Autodesk Inventor part; units mm, degrees
ref_plane "YZ Plane" through (0, 0, 0) normal (1, 0, 0) x (0, 1, 0)
ref_plane "XZ Plane" through (0, 0, 0) normal (0, 1, 0) x (-1, 0, 0)
ref_plane "XY Plane" through (0, 0, 0) normal (0, 0, 1) x (1, 0, 0)
sketch "Sketch1" plane through (0, 0, 0) normal (0, 1, 0) x (-1, 0, 0)
  circle A0 centre (0, 0) radius 13.95
  line L0 (-1.48, 13.8713) -> (-1.48, 10.9113) construction
  line L1 (-1.48, 10.9113) -> (1.48, 10.9113) construction
  line L2 (1.48, 10.9113) -> (1.48, 13.8713) construction
  line L3 (1.33, 13.8865) -> (1.33, 11.0613)
  line L4 (1.33, 11.0613) -> (-1.33, 11.0613)
  line L5 (-1.33, 11.0613) -> (-1.33, 13.8865)
  line L6 (-1.33, -13.8865) -> (-1.33, -11.0613)
  line L7 (-1.33, -11.0613) -> (1.33, -11.0613)
  line L8 (1.33, -11.0613) -> (1.33, -13.8865)
  arc A1 (15.7257, 8.6547) -> (8.6547, -15.7257) centre (0, 0) ccw
  line L9 (0, 0) -> (0, -53.8283) construction
  line L10 (0, 0) -> (-28.2843, -28.2843) construction
  line L11 (0, 0) -> (-45.9619, 45.9619) construction
  line L12 (0, 0) -> (-69.2668, 0) construction
  circle A2 centre (-28.2843, -28.2843) radius 3
  circle A3 centre (-45.9619, 45.9619) radius 3
  line L13 (-8.6547, -15.7257) -> (-24.7487, -31.8198)
  arc A4 (-31.8198, -24.7487) -> (-24.7487, -31.8198) centre (-28.2843, -28.2843) ccw
  line L14 (-31.8198, -24.7487) -> (-15.7257, -8.6547)
  line L15 (-15.7257, 8.6547) -> (-49.4975, 42.4264)
  arc A5 (-49.4975, 49.4975) -> (-49.4975, 42.4264) centre (-45.9619, 45.9619) ccw
  arc A6 (0, 70) -> (-2.9993, 69.9357) centre (0, 0) ccw
  line L16 (0, 70) -> (0, 0) construction
  circle A7 centre (28.2843, -28.2843) radius 3
  circle A8 centre (45.9619, 45.9619) radius 3
  line L17 (8.6547, -15.7257) -> (24.7487, -31.8198)
  arc A9 (24.7487, -31.8198) -> (31.8198, -24.7487) centre (28.2843, -28.2843) ccw
  line L18 (31.8198, -24.7487) -> (15.7257, -8.6547)
  line L19 (15.7257, 8.6547) -> (49.4975, 42.4264)
  arc A10 (49.4975, 42.4264) -> (49.4975, 49.4975) centre (45.9619, 45.9619) ccw
  arc A11 (49.4975, 49.4975) -> (4.9968, 69.8214) centre (0, 0) ccw
  arc A12 (15.7257, -8.6547) -> (15.7257, 8.6547) centre (0, 0) ccw
  arc A13 (8.6547, -15.7257) -> (15.7257, -8.6547) centre (0, 0) ccw
  circle A14 centre (0, 70) radius 3
  circle A15 centre (0, 70) radius 5
  arc A16 (-2.9993, 69.9357) -> (-4.9968, 69.8214) centre (0, 0) ccw
  arc A17 (2.9993, 69.9357) -> (0, 70) centre (0, 0) ccw
  arc A18 (4.9968, 69.8214) -> (2.9993, 69.9357) centre (0, 0) ccw
  arc A19 (-4.9968, 69.8214) -> (-49.4975, 49.4975) centre (0, 0) ccw
  point P0 (0, 10.9113)
  point P1 (0, 11.0613)
  dimension "d0" = 27.9
  dimension "d1" = 2.96
  dimension "d2" = 2.96
  dimension "d3" = 0.15
  dimension "d4" = 0.15
  dimension "d5" = 0.15
  dimension "d7" = 4
  dimension "d8" = 45
  dimension "d9" = 45
  dimension "d10" = 40
  dimension "d11" = 65
  dimension "d12" = 6
  dimension "d13" = 6
  dimension "d14" = 5
  dimension "d15" = 5
  dimension "d17" = 6
  dimension "d18" = 10
extrude "Extrusion1" add sketch "Sketch1" along normal blind 2.5 contours A12 A13 A1 | A1 L15 A5 A19 A15 A11 A10 L19 | L18 A9 L17 A13 | A1 L13 A4 L14 | A18 A14 A16 A15 | A15 A16 A14 A18
extrude "Extrusion2" add sketch "Sketch1" along normal blind 5 contours L3 L4 L5 A0 | A0 L6 L7 L8
sketch "Sketch2" plane through (0, 5, 0) normal (0, 1, 0) x (1, 0, 0)
  circle A0 centre (0, -8.465) radius 0.915
  line L0 (-1.33, -11.0613) -> (-1.33, -13.8865)
  arc A1 (-1.33, -13.8865) -> (1.33, -13.8865) centre (0, 0) ccw
  line L1 (1.33, -13.8865) -> (1.33, -11.0613)
  line L2 (1.33, -11.0613) -> (-1.33, -11.0613)
  circle A2 centre (0, -8.465) radius 2.9171
  dimension "d23" = 1.83
  dimension "d24" = 8.465
extrude "Extrusion3" add sketch "Sketch2" along normal blind 2
mirror "Mirror1" about plane through (0, 0, 0) normal (0, 0, 1) of "Extrusion3"
properties part number "Pok Y-Carriage" material "ABS Plastic"
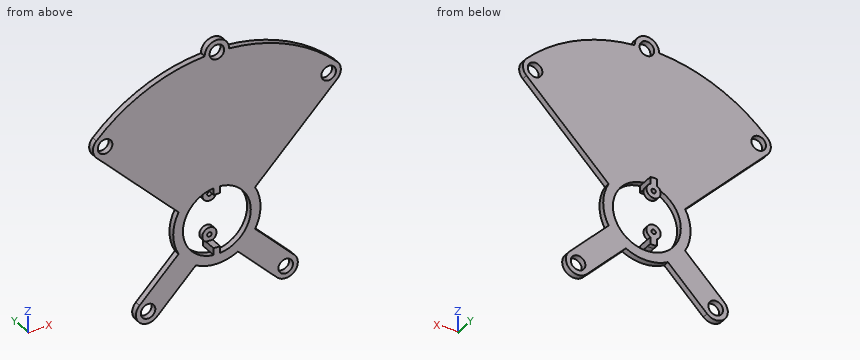
CAD build for the part. Positions are in the model's coordinates, mm. Give positions to 0.01 mm unless a question says otherwise; leave off trailing zeros. Loops run counter-clockwise (first coordinate to the right, second up) from the corner with the lowest first, then second, coordinate; pieces in that order, holes last. Notation, with made-up numbers: M 84,73.5 L 102,73.5 A27 ccw 102,101.5 Z; hole C 57.25,55 d9. An arc over 180 degrees is marked long. One line per question, with ' | ' between items. Start each with the question number.
1. Saw through at D-D on z = 62.5. Give the cut face in (x, y).
2. Saw through at A-A on y = 3.75. Give the cut face in (x, z).
3. Flat gauge pins, fed straight in: pin 1 (0.8 mm diameter, centred on x = -0.5, y = 1.5, fed in from -Z); pin 2 (12 mm diameter, centred on x = 24.5, z = 32.5, fed in from +Y); pin 3 (1.4 mm diameter, centred on y = 3, z = 12, fed in from +X). Where does each tip first touch, or does it go through?
4. Saw through at C-C on z = 40.5. Give the cut face in (x, y).
5. Saw through at B-B on z = 0. Give the cut face in (x, y), plus the area to 3 significant figures.
6. Probe L1, parallel to Z at x = 0, y = 6.3; L2, parallel to X at y = 1.5, z = 70; L3, parallel to X at y = 5.25, z = -8. List the from-to ranges inside material, lowest first. Write a range as from..to.
Result sheet:
1) outline: M -31.52,0 L 31.52,0 L 31.52,2.5 L -31.52,2.5 Z
2) outline: M -1.33,-13.89 A13.95 ccw 1.33,-13.89 L 1.33,-11.06 L -1.33,-11.06 Z; M -1.33,11.06 L 1.33,11.06 L 1.33,13.89 A13.95 ccw -1.33,13.89 Z
3) pin 1: stops at z = -17.95 | pin 2: stops at y = 2.5 | pin 3: stops at x = 19.56
4) outline: M -47.57,0 L 47.57,0 L 47.57,2.5 L -47.57,2.5 Z
5) outline: M -17.95,0 L -13.95,0 L -13.95,2.5 L -17.95,2.5 Z; M 13.95,0 L 17.95,0 L 17.95,2.5 L 13.95,2.5 Z | area: 20.0 mm^2
6) L1: z = -13.95..-9.38, -7.55..-5.55, 5.55..7.55, 9.38..13.95 | L2: x = -5..-3, 3..5 | L3: x = -2.88..-0.79, 0.79..2.88
